Autodesk Inventor part; units mm, degrees
ref_plane "YZ Plane" through (0, 0, 0) normal (1, 0, 0) x (0, 1, 0)
ref_plane "XZ Plane" through (0, 0, 0) normal (0, 1, 0) x (-1, 0, 0)
ref_plane "XY Plane" through (0, 0, 0) normal (0, 0, 1) x (1, 0, 0)
sketch "Szkic8" plane through (0, 0, 0) normal (0, 1, 0) x (-1, 0, 0)
  circle A0 centre (0, 0) radius 52
  circle A1 centre (0, 0) radius 50.5
  dimension "d53" = 104
  dimension "d54" = 1.5
extrude "Wyciągnięcie proste2" add sketch "Szkic8" along normal mid plane 200
sketch "Szkic13" plane through (0, 0, 0) normal (0, 0, 1) x (1, 0, 0)
  circle A0 centre (0, 0) radius 14.5
  circle A1 centre (0, 0) radius 13
  dimension "d67" = 29
  dimension "d68" = 1.5
extrude "Wyciągnięcie proste6" add sketch "Szkic13" along normal blind 53.5
sketch "Szkic14" plane through (0, 0, 53.5) normal (0, 0, 1) x (1, 0, 0)
  circle A0 centre (0, 0) radius 13
extrude "Wyciągnięcie proste7" cut sketch "Szkic14" against normal blind 53.5
sketch "Szkic15" plane through (0, -100, 0) normal (0, -1, 0) x (1, 0, 0)
  circle A0 centre (0, 0) radius 50.5
extrude "Wyciągnięcie proste8" cut sketch "Szkic15" against normal blind 200
fillet "Zaokrąglenie3" radius 1.5 2 edges at (0, 14.5, 52) (0, -14.5, 52)
fillet "Zaokrąglenie4" radius 3 2 edges at (-0.0027, -13, 50.5) (0, 13, 50.5)
equation "\"d53\" = OD"
equation "\"d54\" = THK"
equation "\"d55\" = L1"
equation "\"d67\" = OD2"
equation "\"d68\" = THK"
equation "\"d69\" = L2"
equation "\"d71\" = L2"
equation "\"d73\" = L1"
equation "\"d75\" = THK"
equation "\"d76\" = 2 * THK"
equation "\"SzerokośćGięciaPodcięcia\" = Grubość"
equation "\"RozmiarPodcięciaNarożnika\" = 4 * Grubość"
equation "\"PromieńPrzejścia\" = PromieńGięcia"
equation "\"Rozmiar_promienia_Jacobiego\" = PromieńGięcia"
equation "\"Wielk_odstępu\" = Grubość"
equation "\"d2\" = PromieńGięcia"
equation "\"d23\" = PromieńGięcia"
equation "\"OD\" = 104"
equation "\"THK\" = 1.5"
equation "\"L1\" = 200"
equation "\"L2\" = 53.5"
equation "\"OD2\" = 29"
properties part number "Trójnik red. krótki  Ø104 29 104 s=1,5 L=200" material "304"
Build history of the part. All positions in model axes, mm. A direction names the side the tool comes from. Coordinates: 2 decimals unless noted, no trailing zeros. Order: outer loops, then holes, each group sorted by start corner. A loop starts at its lowest first (then second) coordinate and runs counter-clockwise, first axis right, second up. Notation, with made-up numbers: (38, 85.5) -> (91, 85.5) arc R15 cw to (91, 110.5) -> close; hole circle Ø4 at (46.5, 77.5). An arc over 180 degrees is marked (long way). Answer in a Markdown table with one row per item. Add a question column.
Q1. Which spindle directions (+Z, -Z, +X, -X, +Y, -Y) get a long thin tool onto all of the face, cutting with end or side? Do faces 4 (the face through (27, -100, 43)), 5 (the face through (7.795, -12.226, 53.077)). Say none if no direction does.
Q2. Band-saw the part on A-A, the plane z = 0. List the corners of the cut face in (x, y).
Q3. Wall check: line 1 along Z through (x, y) = (0, -55); line 2 along Z through (x, y) = (24.5, -39); line 3 along X through (y, z) = (0, 51.9). Give the ranges that are in metal, low to high. Write a range as [from, to].
Q4. Drop flat-ended pins along their axis: pin 1 (1 mm diameter, centred on x = 22.5, y = -28, fed in from +Z); pin 2 (15.5 mm diameter, centred on x = 0, y = 0, fed in from +Z); pin 3 (12 mm diameter, centred on x = -11, y = 77, fed in from +Z). Give the stop position or say it passes through.
Q5. Mould opens along X. For faces 1 (the face through (-9, 10, 53.5)), 2 (the face through (6.769, -1.4, -51.557)), 3 (the face through (10.95, 1.4, -49.3)) say: +X half, -X half, draft (parallel to the pull), parting line (faces both ways), or undercut.
Q6. Band-saw the part on C-C, the plane y = 28.5. List the corners of the cut face in (x, z).
Answers follow:
| question | item | result |
|---|---|---|
| 1 | face 4 | +Z, -Z, +X, -X, -Y |
| 1 | face 5 | +Z |
| 2 | outline | (-52, -100) -> (-50.5, -100) -> (-50.5, 100) -> (-52, 100) -> close; (50.5, -100) -> (52, -100) -> (52, 100) -> (50.5, 100) -> close |
| 3 | line 1 | [-52, -50.5], [50.5, 52] |
| 3 | line 2 | [-45.87, -44.16], [44.16, 45.87] |
| 3 | line 3 | [-14.5, -13], [13, 14.5] |
| 4 | pin 1 | z = 47.12 |
| 4 | pin 2 | z = -49.9 |
| 4 | pin 3 | z = 51.76 |
| 5 | face 1 | draft |
| 5 | face 2 | parting line |
| 5 | face 3 | undercut |
| 6 | outline | circle Ø104 at (0, 0); hole circle Ø101 at (0, 0) |
